Work out the finished part from the listing and answer in its coordinate system (mm). A direction names the side the tool comes from. Round coordinates to 2 decimals unless told otherwise and drop trailing zeros. Order: outer loops, then holes, each group sorted by start corner. A loop starts at its lowest first (then second) coordinate and runs counter-clockwise, first axis right, second up. Notation, with made-up numbers: (2, 45.5) -> (29, 45.5) arc R13 cw to (29, 59.5) -> close; hole circle Ø8 at (59.25, -1). An arc over 180 degrees is marked (long way). Use a Markdown table: item, result. Add a question column.
Item 1: Find the intervals of material crossed by L1, parallel to Z at x = 8257, y = 3007.5; L2, parallel to X at y = 2993, z = -5.75; L3, parallel to X at y = 2984, z = -9, in increasing order. Write a range as [from, to].
Item 2: A cutting plane is placed at D-D, the plane y = 2987.5. Determine the outline of the cut face in (x, z), plus the area to 3 significant figures.
Item 3: Flat-ended cylindrical pins translate along their axes: P1, Ø2, axis at x = 8237.5, y = 3001, coming from the -Z side; P2, Ø1, axis at x = 8235, z = 2.5, coming from the -Y side; P3, Ø5, axis at x = 8236.97, y = 3008.37, coming from the -Z side; P4, Ø6, axis at x = 8220, z = -15.5, coming from the +Y side. Find the tip coordinate at first contact, or state that the pin passes through.
Item 4: For a pull along Y with two mould halves and no side action, classify faces 5 (the flat face through (8237, 3002, 1)), 6 (the flat face through (8225, 2993.613, -10)), 7 (the flat face through (8237, 3005, 0)), 8 (the flat face through (8222.13, 2988.26, 1.48)) as +Y half, -Y half, draft (parallel to the pull), parting line (faces both ways), or undercut.
Item 5: A cutting plane is placed at A-A, the plane y = 2999. Determine the outline of the cut face in (x, z).
Item 6: A tool of negligible diameter and unlimited length cuts with its end or side. For faces 1 (the flat face through (8237, 2990, 1)), 2 (the flat face through (8249, 2993.613, -10)), 3 (the flat face through (8214.671, 3003, 1)), 4 (the flat face through (8237, 2993.613, 2)), from which of +Z, -Z, +X, -X, +Y, -Y can it reach the whole face along a straight path? Write none if from no direction.
Item 7: A cutting plane is placed at C-C, the plane z = 1.5. Determine the outline of the cut face in (x, y).
Item 8: A cutting plane is placed at B-B, the plane x = 8252. Determine the outline of the cut face in (y, z).
from build123d import *

# Parameters (mm, degrees)
SKETCH_2_R      = 10.5
SKETCH_2_R_2    = 2.2
EXTRUDE_1_DEPTH = 3
EXTRUDE_START   = -2
EXTRUDE_3_DEPTH = 2
EXTRUDE_START_2 = 20
EXTRUDE_5_DEPTH = 20


with BuildPart() as part:
    # 草图2 → 凸台-拉伸1 (new body)
    with BuildSketch(Plane.XY):
        with BuildLine():
            Line((8214.670798087, 3013.113410171), (8259.670798087, 3013.113410171))
            Line((8259.670798087, 3013.113410171), (8259.670798087, 2993.613410171))
            Line((8259.670798087, 2993.613410171), (8244.413270011, 2982.956276447))
            ThreePointArc((8244.413270011, 2982.956276447), (8236.88707696, 2980.614241973), (8229.391164024, 2983.051452794))
            Line((8229.391164024, 2983.051452794), (8214.670798087, 2993.613410171))
            Line((8214.670798087, 2993.613410171), (8214.670798087, 3013.113410171))
        make_face()
        with Locations((8236.969436473, 2993.613410171)):
            Circle(SKETCH_2_R, mode=Mode.SUBTRACT)
        with Locations((8236.969436473, 3008.366275847)):
            Circle(SKETCH_2_R_2, mode=Mode.SUBTRACT)
        with Locations((8221.719436473, 3009.366275847)):
            Circle(SKETCH_2_R_2, mode=Mode.SUBTRACT)
        with Locations((8252.219436473, 3009.366275847)):
            Circle(SKETCH_2_R_2, mode=Mode.SUBTRACT)
    extrude(amount=EXTRUDE_1_DEPTH)

    # 草图3 → 凸台-拉伸3 (add)
    with BuildSketch(Plane.XY.offset(3).offset(EXTRUDE_START)):
        with BuildLine():
            Line((8247.469436473, 2993.613410171), (8226.469436473, 2993.613410171))
            ThreePointArc((8226.469436473, 2993.613410171), (8236.969436473, 2983.113410171), (8247.469436473, 2993.613410171))
        make_face()
        with BuildLine():
            Line((8228.607869965, 2999.9643318), (8245.331002981, 2999.9643318))
            ThreePointArc((8245.331002981, 2999.9643318), (8236.969436473, 3004.113410171), (8228.607869965, 2999.9643318))
        make_face()
    extrude(amount=EXTRUDE_3_DEPTH)

    # 草图5 → 凸台-拉伸5 (add)
    with BuildSketch(Plane(origin=(0, 0, 0), x_dir=(-1, 0, 0), z_dir=(0, 0, -1)).offset(EXTRUDE_START_2)):
        with BuildLine():
            Line((-8247.469436473, 2993.613410171), (-8249.968865573, 2993.613410171))
            ThreePointArc((-8249.968865573, 2993.613410171), (-8236.969436473, 2980.61398107), (-8223.970007373, 2993.613410171))
            Line((-8223.970007373, 2993.613410171), (-8226.469436473, 2993.613410171))
            ThreePointArc((-8226.469436473, 2993.613410171), (-8236.969436473, 2983.113410171), (-8247.469436473, 2993.613410171))
        make_face()
    extrude(amount=-EXTRUDE_5_DEPTH)


solid = part.part
Reported:
| question | item | result |
|---|---|---|
| 1 | L1 | [0, 3] |
| 1 | L2 | [8223.98, 8226.49], [8247.45, 8249.95] |
| 1 | L3 | [8228.22, 8232.75], [8241.19, 8245.72] |
| 2 | outline | (8223.19, 0) -> (8225.5, 0) -> (8225.5, -20) -> (8228.43, -20) -> (8228.43, 1) -> (8245.51, 1) -> (8245.51, -20) -> (8248.44, -20) -> (8248.44, 0) -> (8250.92, 0) -> (8250.92, 3) -> (8223.19, 3) -> close |
| 2 | area | 184 mm² |
| 3 | P1 | z = 1 |
| 3 | P2 | y = 2980.7 |
| 3 | P3 | z = 0 |
| 3 | P4 | through |
| 4 | face 5 | undercut |
| 4 | face 6 | +Y half |
| 4 | face 7 | draft |
| 4 | face 8 | -Y half |
| 5 | outline | (8214.67, 0) -> (8227.96, 0) -> (8227.96, 3) -> (8214.67, 3) -> close; (8245.98, 0) -> (8259.67, 0) -> (8259.67, 3) -> (8245.98, 3) -> close |
| 6 | face 1 | -Z |
| 6 | face 2 | -Z, +X, -X, +Y |
| 6 | face 3 | +Z, -Z, -X, +Y, -Y |
| 6 | face 4 | +Z, -Z |
| 7 | outline | (8214.67, 2993.61) -> (8229.39, 2983.05) arc R13 ccw to (8244.41, 2982.96) -> (8259.67, 2993.61) -> (8259.67, 3013.11) -> (8214.67, 3013.11) -> close; hole circle Ø4.4 at (8221.72, 3009.37); hole (8226.47, 2993.61) -> (8247.47, 2993.61) arc R10.5 ccw to (8245.33, 2999.96) -> (8228.61, 2999.96) arc R10.5 ccw to start; hole circle Ø4.4 at (8236.97, 3008.37); hole circle Ø4.4 at (8252.22, 3009.37) |
| 8 | outline | (2988.26, 0) -> (3007.18, 0) -> (3007.18, 3) -> (2988.26, 3) -> close; (3011.56, 0) -> (3013.11, 0) -> (3013.11, 3) -> (3011.56, 3) -> close |
